Part model, mm, in its own coordinate system. Face numbers are marked on the shaded views. Give positions to 0.01 mm unless a question says otherwise; leave off trailing zeros. Write each loop counter-clockwise with the first axis right and the second up, starting at its lowest first coordinate (ties: lowest second). Pieces come first, ordered by that corner, then holes. Notation, with made-up numbers: (41, 58) - (53, 58) arc R21 cw to (53, 62) - close; hole circle Ø2 at (13.5, 15.5). An arc over 180 degrees is marked (long way). Answer in a Markdown table with one row per item. Add a question column.
1. Band-saw the part on A-A on x = 11.75. Write the cut outline in (y, z), plus the area to 3 significant figures.
2. Band-saw the part on B-B on z = -6.5. Write the cut outline in (x, y).
3. Band-saw the part on D-D on x = -13.5. Write the cut outline in (y, z), plus the area to 3 significant figures.
4. Pull direction X, two halves, no side cores. Call the marked faces 1, 2, 3 and 4: released by +X, released by -X, zero draft, split by the parting line, or undercut.
5. Band-saw the part on C-C on y = 2.5. Write the cut outline in (x, z).
6. Probe line 1 along X through (y, z) = (0.7, -6.5); line 2 along Z through (x, y) = (-11.75, 2.1); line 3 along X through (y, z) = (1.55, -4.25). List the from-to ranges inside material, lowest first.
```python
from build123d import *

# Parameters (mm, degrees)
ESQUISSE1_W        = 18.25
ESQUISSE1_H        = 13
ESQUISSE1_R        = 2.6
BOSS_EXTRU_1_DEPTH = 3


with BuildPart() as part:
    # Esquisse1 → Boss.-Extru.1 (new body)
    with BuildSketch(Plane(origin=(0, 0, 0), x_dir=(1, 0, 0), z_dir=(0, 1, 0))):
        with Locations((-9.125, 6.5)):
            Rectangle(ESQUISSE1_W, ESQUISSE1_H)
        with Locations((-11.75, 6.5)):
            Circle(ESQUISSE1_R, mode=Mode.SUBTRACT)
    boss_extru_1 = extrude(amount=BOSS_EXTRU_1_DEPTH)

    # Symétrie1: Boss.-Extru.1 across plane
    add(boss_extru_1.mirror(Plane(origin=(0, 0, 0), x_dir=(0, 0, 1), z_dir=(1, 0, 0))))


solid = part.part
```
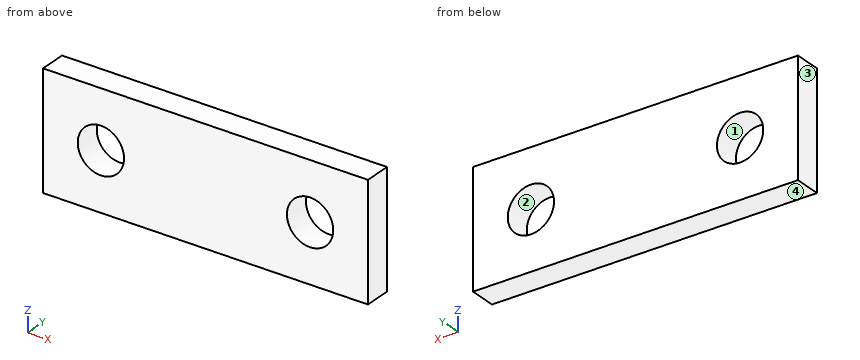
Values:
| question | item | result |
|---|---|---|
| 1 | outline | (0, -13) - (3, -13) - (3, -9.1) - (0, -9.1) - close; (0, -3.9) - (3, -3.9) - (3, 0) - (0, 0) - close |
| 1 | area | 23.4 mm² |
| 2 | outline | (-18.25, 0) - (-14.35, 0) - (-14.35, 3) - (-18.25, 3) - close; (-9.15, 0) - (9.15, 0) - (9.15, 3) - (-9.15, 3) - close; (14.35, 0) - (18.25, 0) - (18.25, 3) - (14.35, 3) - close |
| 3 | outline | (0, -13) - (3, -13) - (3, -8.42) - (0, -8.42) - close; (0, -4.58) - (3, -4.58) - (3, 0) - (0, 0) - close |
| 3 | area | 27.5 mm² |
| 4 | face 1 | undercut |
| 4 | face 2 | undercut |
| 4 | face 3 | released by -X |
| 4 | face 4 | zero draft |
| 5 | outline | (-18.25, -13) - (18.25, -13) - (18.25, 0) - (-18.25, 0) - close; hole circle Ø5.2 at (-11.75, -6.5); hole circle Ø5.2 at (11.75, -6.5) |
| 6 | line 1 | x = -18.25 to -14.35, -9.15 to 9.15, 14.35 to 18.25 |
| 6 | line 2 | z = -13 to -9.1, -3.9 to 0 |
| 6 | line 3 | x = -18.25 to -13.05, -10.45 to 10.45, 13.05 to 18.25 |
